from build123d import *

# Parameters (mm, degrees)
IZIM1_R                     = 2.35
IZIM1_R_2                   = 0.5
Y_KSEKLIK_EKSTR_ZYON1_DEPTH = 1.5
IZIM1_3_R                   = 2.35
IZIM1_3_R_2                 = 1.275
Y_KSEKLIK_EKSTR_ZYON2_DEPTH = 0.5
IZIM2_R                     = 3.45
IZIM2_R_2                   = 2.3
Y_KSEKLIK_EKSTR_ZYON3_DEPTH = 2.5
RADYUS1_R                   = 0.1


with BuildPart() as part:
    # izim1 → Y_kseklik-Ekstr_zyon1 (new body)
    with BuildSketch(Plane(origin=(0, 0, 0), x_dir=(1, 0, 0), z_dir=(0, 1, 0))):
        with BuildLine():
            Line((1.9, 2.9), (1.9, 6.75))
            ThreePointArc((1.9, 6.75), (0, 8.65), (-1.9, 6.75))
            Line((-1.9, 6.75), (-1.9, 3.45))
            Line((-1.9, 3.45), (-16.894677741, 1.487313207))
            ThreePointArc((-16.894677741, 1.487313207), (-18.2, 0), (-16.894677741, -1.487313207))
            Line((-16.894677741, -1.487313207), (-1.9, -3.45))
            Line((-1.9, -3.45), (-1.9, -6.75))
            ThreePointArc((-1.9, -6.75), (0, -8.65), (1.9, -6.75))
            Line((1.9, -6.75), (1.9, -2.9))
            Line((1.9, -2.9), (14.862072923, -1.491218417))
            ThreePointArc((14.862072923, -1.491218417), (16.2, 0), (14.862072923, 1.491218417))
            Line((14.862072923, 1.491218417), (1.9, 2.9))
        make_face()
        Circle(IZIM1_R, mode=Mode.SUBTRACT)
        with Locations((-16.7, 0)):
            Circle(IZIM1_R_2, mode=Mode.SUBTRACT)
        with Locations((-14.7, 0)):
            Circle(IZIM1_R_2, mode=Mode.SUBTRACT)
        with Locations((-12.7, 0)):
            Circle(IZIM1_R_2, mode=Mode.SUBTRACT)
        with Locations((-10.7, 0)):
            Circle(IZIM1_R_2, mode=Mode.SUBTRACT)
        with Locations((-8.7, 0)):
            Circle(IZIM1_R_2, mode=Mode.SUBTRACT)
        with Locations((-6.7, 0)):
            Circle(IZIM1_R_2, mode=Mode.SUBTRACT)
        with Locations((-4.7, 0)):
            Circle(IZIM1_R_2, mode=Mode.SUBTRACT)
        with Locations((14.7, 0)):
            Circle(IZIM1_R_2, mode=Mode.SUBTRACT)
        with Locations((12.7, 0)):
            Circle(IZIM1_R_2, mode=Mode.SUBTRACT)
        with Locations((10.7, 0)):
            Circle(IZIM1_R_2, mode=Mode.SUBTRACT)
        with Locations((8.7, 0)):
            Circle(IZIM1_R_2, mode=Mode.SUBTRACT)
        with Locations((6.7, 0)):
            Circle(IZIM1_R_2, mode=Mode.SUBTRACT)
        with Locations((4.7, 0)):
            Circle(IZIM1_R_2, mode=Mode.SUBTRACT)
        with Locations((0, 6.7)):
            Circle(IZIM1_R_2, mode=Mode.SUBTRACT)
        with Locations((0, 4.7)):
            Circle(IZIM1_R_2, mode=Mode.SUBTRACT)
        with Locations((0, -6.7)):
            Circle(IZIM1_R_2, mode=Mode.SUBTRACT)
        with Locations((0, -4.7)):
            Circle(IZIM1_R_2, mode=Mode.SUBTRACT)
    extrude(amount=Y_KSEKLIK_EKSTR_ZYON1_DEPTH)

    # izim1_3 → Y_kseklik-Ekstr_zyon2 (add)
    with BuildSketch(Plane(origin=(0, 0, 0), x_dir=(1, 0, 0), z_dir=(0, 1, 0))):
        Circle(IZIM1_3_R)
        Circle(IZIM1_3_R_2, mode=Mode.SUBTRACT)
    extrude(amount=Y_KSEKLIK_EKSTR_ZYON2_DEPTH)

    # izim2 → Y_kseklik-Ekstr_zyon3 (add)
    with BuildSketch(Plane.XZ):
        Circle(IZIM2_R)
        Circle(IZIM2_R_2, mode=Mode.SUBTRACT)
    extrude(amount=Y_KSEKLIK_EKSTR_ZYON3_DEPTH)

    # Radyus1
    radyus1_edges = [part.edges().sort_by_distance(p)[0] for p in [
        (1.9, 0.75, -2.9),
        (1.9, 0.75, 2.9),
        (-1.9, 0.75, 3.45),
        (-1.9, 0.75, -3.45),
    ]]
    fillet(radyus1_edges, radius=RADYUS1_R)


solid = part.part
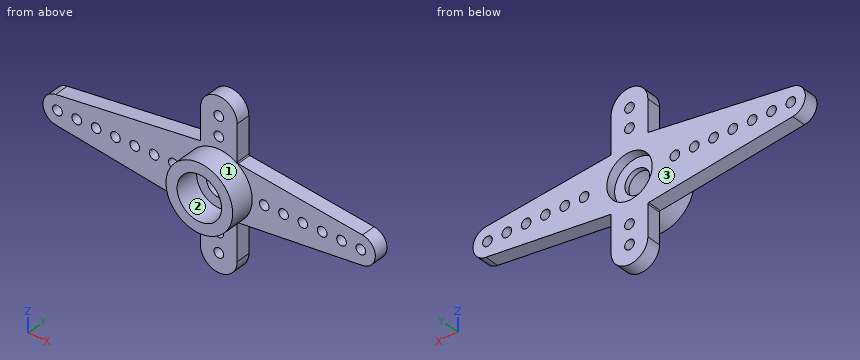
Source: CAD feature listing. Evaluate the final solid. Frame: model axes, mm. Face numbers are marked on the shaded views. Coordinates: 2 decimals unless noted, no trailing zeros. Loops run counter-clockwise (first coordinate to the right, second up) from the corner with the lowest first, then second, coordinate; pieces in that order, holes last. Notation, with made-up numbers: (36, 43.25) - (92, 43.25) arc R24 ccw to (92, 62.25) - close; hole circle Ø11 at (86.25, -14). An arc over 180 degrees is marked (long way). One line per item, written item: value. Start each with the question number.
1. Mould query, pull axis X, two halves, no side actions, for the marked faces 1, 2 and 3. Classes: pulls with the +X half, pulls with the -X half, needs draft (parallel to the pull), parting line crosses it, or undercut.
2. Ray query, L1, parallel to Z at x = 0, y = 0.45 (3 decimals); L2, parallel to X at y = 0.5, z = 4.7; L3, parallel to Z at x = -10.7, y = 0.7. Return the intervals inside material, ascending.
3. Section C-C (y = -1.9). Return the cut outline in (x, z), and give its area (3 significant figures).
4. Section A-A (z = 4.7). Return the cut outline in (x, y), and give its area (3 significant figures).
5. Section B-B (x = 6.7). Return the cut outline in (y, z).
6. Contact query for flat-ended pins moving along their axis: P1, Ø0.8, axis at y = 1, z = -5, coming from the -X side; P2, Ø3, axis at x = 0, z = 0, coming from the -Y side; P3, Ø1.2, axis at y = 0.5, z = -4, coming from the +X side. Output: stop coordinate, or through.
Verdict:
1. face 1: parting line crosses it
1. face 2: undercut
1. face 3: needs draft
2. L1: z = -8.65 to -7.2, -6.2 to -5.2, -4.2 to -1.275, 1.275 to 4.2, 5.2 to 6.2, 7.2 to 8.65
2. L2: x = -1.9 to -0.5, 0.5 to 1.9
2. L3: z = -2.3 to -0.5, 0.5 to 2.3
3. outline: circle Ø6.9 at (0, 0); hole circle Ø4.6 at (0, 0)
3. area: 20.8 mm2
4. outline: (-1.9, 0) - (-0.5, 0) - (-0.5, 1.5) - (-1.9, 1.5) - close; (0.5, 0) - (1.9, 0) - (1.9, 1.5) - (0.5, 1.5) - close
4. area: 4.20 mm2
5. outline: (0, -2.38) - (1.5, -2.38) - (1.5, -0.5) - (0, -0.5) - close; (0, 0.5) - (1.5, 0.5) - (1.5, 2.38) - (0, 2.38) - close
6. P1: stops at x = -1.9
6. P2: stops at y = 0
6. P3: stops at x = 1.9
